```python
from build123d import *

# Parameters (mm, degrees)
F0_R     = 1.7145
F1_DEPTH = 3.175


with BuildPart() as f1:
    # F0 (on Front) → F1 (new body)
    with BuildSketch(Plane.XZ):
        Polygon((73.120295, 17.4625), (-79.279705, 17.4625), (-79.279705, 0), (-60.229705, 0), (-60.229705, -1.5875), (35.020295, -1.5875), (35.020295, 0), (47.720295, 0), (73.120295, 0), align=None)
        with Locations((-55.149705, 10.8331)):
            Circle(F0_R, mode=Mode.SUBTRACT)
        Polygon((-60.229705, -3.175), (-79.279705, -3.175), (-79.279705, -20.6375), (73.120295, -20.6375), (73.120295, -3.175), (47.720295, -3.175), (35.020295, -3.175), (35.020295, -1.5875), (-60.229705, -1.5875), align=None)
    extrude(amount=F1_DEPTH)


solid = f1.part
```
Geometry check sheet. Reference: the model listing, model coordinates, mm. A direction names the side the tool comes from. Round coordinates to 2 decimals unless told otherwise and drop trailing zeros. Order: outer loops, then holes, each group sorted by start corner. A loop starts at its lowest first (then second) coordinate and runs counter-clockwise, first axis right, second up. Notation, with made-up numbers: (-34.75, 59) -> (-10.75, 59) arc R13 cw to (-10.75, 76) -> close; hole circle Ø11 at (11.5, 75). An arc over 180 degrees is marked (long way). Return JSON: item names as keys, results as strings. Group by question number.
Q1. Gauge pin test, flat end, axial feed: pin 1 (1 mm diameter, centred on y = -2, z = -1.5, fed in from -X). Record the tip position at first contact, or that the pin passes through.
Q2. Tool access check on faces 4 (the flat face through (-79.28, -2, -12)), 5 (the flat face through (-60.23, -2, -2)), 6 (the flat face through (54, -2, -3.175)). Record the directions out of +Z, -Z, +X, -X, +Y, -Y that give a thin tool (end or side, any length) a straight path to the whole face; none if there is none.
Q3. Release check for a two-part mould opening along X. For faces 1 (the flat face through (54, -2, 0)), 2 (the flat face through (35.02, -2, -2)), 3 (the cylindrical face through (-56.51, -1.57, 9.79)) record: released by +X, released by -X, zero draft, split by the parting line, or undercut.
Q4. Section check A-A, the plane y = -1.5. Record the boundary of the cut face in (x, z) (1 decimal), plus the area to 3 significant figures.
Q5. Material ranges on probe 1 along Z at (x, y) = (52.5, -2.25) (1 decimal); probe 2 along X at (y, z) = (-2.3, -1); probe 3 along X at (y, z) = (-2.25, 9.5), recorded low to high. Write a range as from..to.
Numbers:
{
 "1": {"pin 1": "x = -60.23"},
 "2": {"face 4": "+Z, -Z, -X, +Y, -Y", "face 5": "-X, +Y, -Y", "face 6": "+X, +Y, -Y"},
 "3": {"face 1": "zero draft", "face 2": "released by +X", "face 3": "undercut"},
 "4": {"outline": "(-79.3, -20.6) -> (73.1, -20.6) -> (73.1, -3.2) -> (35, -3.2) -> (35, 0) -> (73.1, 0) -> (73.1, 17.5) -> (-79.3, 17.5) -> (-79.3, 0) -> (-60.2, 0) -> (-60.2, -3.2) -> (-79.3, -3.2) -> close; hole circle Ø3.4 at (-55.1, 10.8)", "area": "5,620 mm^2"},
 "5": {"probe 1": "-20.6..-3.2, 0..17.5", "probe 2": "-60.23..35.02", "probe 3": "-79.28..-56.23, -54.07..73.12"}
}
